Job drawing, mm, ordinate dimensions from the low corner. One solid piece. Give positions to 0.01 mm unless a question says otherwise; leave off trailing zeros. Write each loop counter-clockwise with the first axis right and the second up, starting at its lowest first coordinate (ties: lowest second). Pieces come first, ordered by that corner, then holes. Notation, with made-up numbers: (-16.5, 89.25) - (6.5, 89.25) arc R8 ccw to (6.5, 100.25) - close; hole circle Ø7 at (46, 1). An arc over 180 degrees is marked (long way). Answer in a Markdown table with one row per item. Add a question column.
1. Band-saw the part on B-B on x = 23.5. Write the cut outline in (y, z).
2. Band-saw the part on A-A on y = 13.5. Write the cut outline in (x, z) (1 decimal).
3. Drop flat-ended pins along their axis: pin 1 Ø1 at (x, y) = (34, 33.5) entering from +Z; pin 2 Ø3 at (y, z) = (31, 31) entering from +X; pin 3 Ø1 at (y, z) = (28.5, 28.5) entering from +X (1 decimal). Give the stop position or say it passes through.
4. Band-saw the part on D-D on x = 33. Write the cut outline in (y, z).
5. Pull direction Z, two halves, no side cores. Call the marked faces 1, 2 and 3: released by +Z, released by -Z, zero draft, split by the parting line, or undercut.
6. Probe line 1 along X through (y, z) = (35.5, 49.5); line 2 along X through (y, z) = (47.5, 34); line 3 along Z through (x, y) = (36, 25.5). List the from-to ranges inside material, lowest first.
7. Band-saw the part on C-C on z = 50. Write the cut outline in (x, y), plus the area to 3 significant figures.
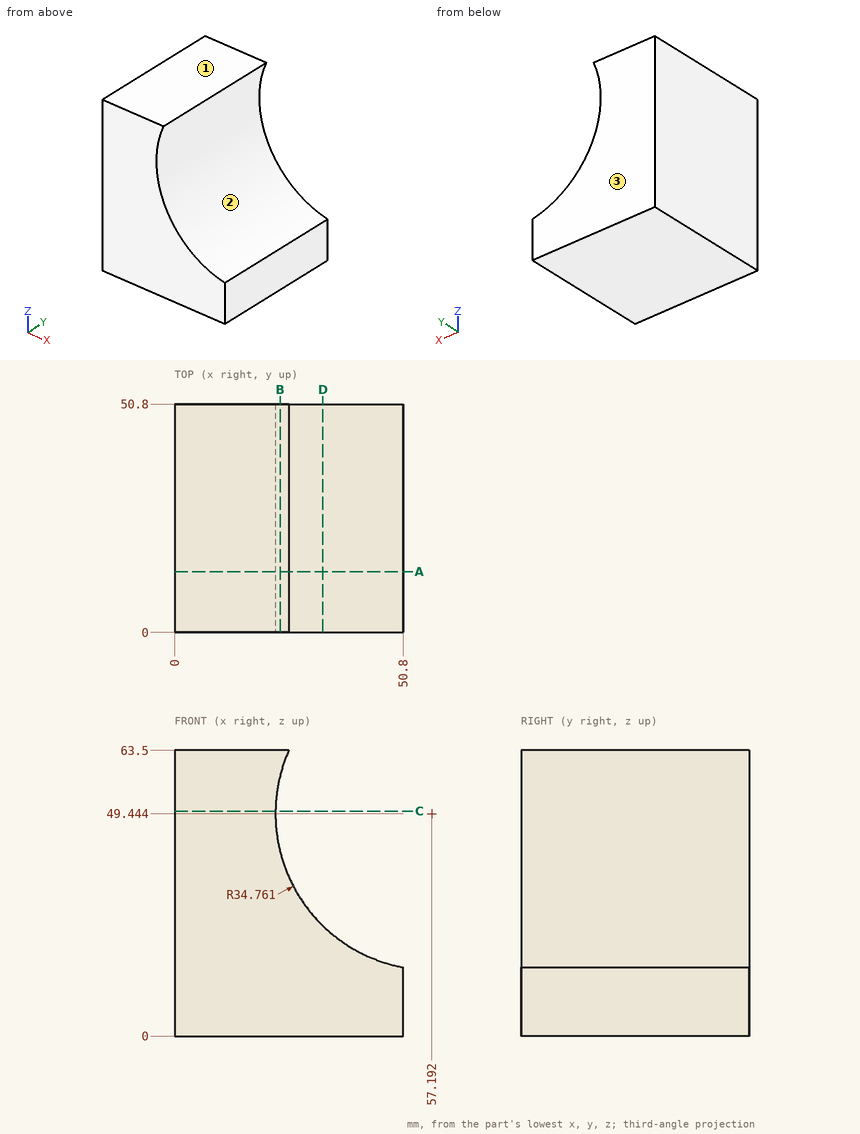
Values:
| question | item | result |
|---|---|---|
| 1 | outline | (0, 0) - (50.8, 0) - (50.8, 40.89) - (0, 40.89) - close; (0, 58) - (50.8, 58) - (50.8, 63.5) - (0, 63.5) - close |
| 2 | outline | (0, 0) - (50.8, 0) - (50.8, 15.3) arc R34.8 cw to (25.4, 63.5) - (0, 63.5) - close |
| 3 | pin 1 | stops at z = 24.01 |
| 3 | pin 2 | stops at x = 28.72 |
| 3 | pin 3 | stops at x = 29.8 |
| 4 | outline | (0, 0) - (50.8, 0) - (50.8, 24.48) - (0, 24.48) - close |
| 5 | face 1 | released by +Z |
| 5 | face 2 | undercut |
| 5 | face 3 | zero draft |
| 6 | line 1 | x = 0 to 22.43 |
| 6 | line 2 | x = 0 to 26.05 |
| 6 | line 3 | z = 0 to 21.89 |
| 7 | outline | (0, 0) - (22.44, 0) - (22.44, 50.8) - (0, 50.8) - close |
| 7 | area | 1,140 mm² |
